from build123d import *
from build123d.topology import SkipClean

# Parameters (mm, degrees)
SKETCH1_W                = 105
SKETCH1_H                = 105
SKETCH1_W_2              = 94
SKETCH1_H_2              = 94
SKETCH1_W_3              = 65
SKETCH1_H_3              = 25
BOSS_EXTRUDE1_DEPTH      = 20
SKETCH2_W                = 65
SKETCH2_H                = 25
SKETCH2_W_2              = 94
SKETCH2_H_2              = 94
BOSS_EXTRUDE2_DEPTH      = 10
SKETCH3_W                = 57
SKETCH3_H                = 26.5
CUT_EXTRUDE1_DEPTH       = 20
SKETCH5_R                = 52.5
BOSS_EXTRUDE4_DEPTH      = 20
SKETCH8_R                = 48.5
CUT_EXTRUDE3_DEPTH       = 107.124926384
BOSS_EXTRUDE5_START      = -38
SKETCH9_R                = 2.5
BOSS_EXTRUDE5_DEPTH      = 12
SKETCH4_R                = 2.5
BOSS_EXTRUDE6_DEPTH      = 20
SKETCH10_W               = 15.5
SKETCH10_H               = 26.597794237
CUT_EXTRUDE4_DEPTH       = 20
BOSS_EXTRUDE8_START      = -45
SKETCH11_R               = 2.5
BOSS_EXTRUDE8_DEPTH      = 15
BOSS_EXTRUDE7_DEPTH      = 20
SKETCH16_R               = 2.5
BOSS_EXTRUDE9_DEPTH      = 30
CUT_EXTRUDE5_START       = -8
CUT_EXTRUDE5_DEPTH       = 8
SKETCH18_R               = 2.5
BOSS_EXTRUDE10_DEPTH     = 12
CUT_EXTRUDE12_DEPTH      = 18
CUT_EXTRUDE12_DEPTH_BACK = 24
CUT_EXTRUDE13_DEPTH      = 15


# Read off the part's stored shape, not the designer's step: Boss-Extrude7
with BuildPart() as part:
    # Sketch1 → Boss-Extrude1 (new body)
    # profile 1 of 2: a face of its own
    with BuildSketch(Plane.XY):
        Rectangle(SKETCH1_W, SKETCH1_H)
        Rectangle(SKETCH1_W_2, SKETCH1_H_2, mode=Mode.SUBTRACT)
    # profile 2 of 2: a face of its own
    with BuildSketch(Plane.XY):
        with Locations((0, -65)):
            Rectangle(SKETCH1_W_3, SKETCH1_H_3)
    extrude(amount=BOSS_EXTRUDE1_DEPTH)

    # Sketch2 → Boss-Extrude2 (add)
    # profile 1 of 3: a face of its own
    with BuildSketch(Plane.XY.offset(20)):
        with Locations((0, -65)):
            Rectangle(SKETCH2_W, SKETCH2_H)
    # profile 2 of 3: a face of its own
    with BuildSketch(Plane.XY.offset(20)):
        Polygon((52.5, 52.5), (-52.5, 52.5), (-52.5, -52.5), (-32.5, -52.5), (32.5, -52.5), (52.5, -52.5), align=None)
        Rectangle(SKETCH2_W_2, SKETCH2_H_2, mode=Mode.SUBTRACT)
    # profile 3 of 3: a face of its own
    with BuildSketch(Plane.XY.offset(20)):
        Rectangle(SKETCH2_W_2, SKETCH2_H_2)
    extrude(amount=BOSS_EXTRUDE2_DEPTH)

    # Sketch3 → Cut-Extrude1 (cut)
    with BuildSketch(Plane(origin=(0, 0, 0), x_dir=(-1, 0, 0), z_dir=(0, 0, -1))):
        with Locations((0, -60.25)):
            Rectangle(SKETCH3_W, SKETCH3_H)
    extrude(amount=-CUT_EXTRUDE1_DEPTH, mode=Mode.SUBTRACT)

    # Sketch5 → Boss-Extrude4 (add)
    with BuildSketch(Plane.XY.offset(30)):
        Circle(SKETCH5_R)
    extrude(amount=BOSS_EXTRUDE4_DEPTH)

    # Sketch8 → Cut-Extrude3 (cut, through all)
    with BuildSketch(Plane.XY.offset(50)):
        Circle(SKETCH8_R)
    extrude(amount=-CUT_EXTRUDE3_DEPTH, mode=Mode.SUBTRACT)

    # Sketch9 → Boss-Extrude5 (add)
    # profile 1 of 3: a face of its own
    with BuildSketch(Plane.XY.offset(50).offset(BOSS_EXTRUDE5_START)):
        with BuildLine():
            Line((57.5, 6.5), (48.5, 6.5))
            Line((48.5, 6.5), (48.5, -6.5))
            Line((48.5, -6.5), (57.5, -6.5))
            ThreePointArc((57.5, -6.5), (64, 0), (57.5, 6.5))
        make_face()
        with Locations((57.5, 0)):
            Circle(SKETCH9_R, mode=Mode.SUBTRACT)
    # profile 2 of 3: a face of its own
    with BuildSketch(Plane.XY.offset(50).offset(BOSS_EXTRUDE5_START)):
        with BuildLine():
            Line((-57.5, 6.5), (-48.5, 6.5))
            Line((-48.5, 6.5), (-48.5, -6.5))
            Line((-48.5, -6.5), (-57.5, -6.5))
            ThreePointArc((-57.5, -6.5), (-64, 0), (-57.5, 6.5))
        make_face()
        with Locations((-57.5, 0)):
            Circle(SKETCH9_R, mode=Mode.SUBTRACT)
    # profile 3 of 3: a face of its own
    with BuildSketch(Plane.XY.offset(50).offset(BOSS_EXTRUDE5_START)):
        with BuildLine():
            Line((-6.5, 57.5), (-6.5, 48.5))
            Line((-6.5, 48.5), (6.5, 48.5))
            Line((6.5, 48.5), (6.5, 57.5))
            ThreePointArc((6.5, 57.5), (0, 64), (-6.5, 57.5))
        make_face()
        with Locations((0, 57.5)):
            Circle(SKETCH9_R, mode=Mode.SUBTRACT)
    extrude(amount=-BOSS_EXTRUDE5_DEPTH)

    # Sketch4 → Boss-Extrude6 (add)
    with BuildSketch(Plane(origin=(0, 0, 0), x_dir=(-1, 0, 0), z_dir=(0, 0, -1))):
        with BuildLine():
            Line((-32.5, -64), (-32.5, -77.5))
            Line((-32.5, -77.5), (32.5, -77.5))
            Line((32.5, -77.5), (32.5, -64))
            Line((32.5, -64), (37.5, -64))
            ThreePointArc((37.5, -64), (42.096194078, -62.096194078), (44, -57.5))
            Line((44, -57.5), (44, -52.5))
            Line((44, -52.5), (52.5, -52.5))
            Line((52.5, -52.5), (52.021296507, -7.073521736))
            ThreePointArc((52.021296507, -7.073521736), (49.206713639, -18.301621043), (44, -28.640006983))
            Line((44, -28.640006983), (44, -20.402205763))
            ThreePointArc((44, -20.402205763), (0, -48.5), (-44, -20.402205763))
            Line((-44, -20.402205763), (-44, -28.640006983))
            ThreePointArc((-44, -28.640006983), (-50.330159944, -14.937369246), (-52.5, 0))
            Line((-52.5, 0), (-52.5, -52.5))
            Line((-52.5, -52.5), (-44, -52.5))
            Line((-44, -52.5), (-44, -57.5))
            ThreePointArc((-44, -57.5), (-42.096194078, -62.096194078), (-37.5, -64))
            Line((-37.5, -64), (-32.5, -64))
        make_face()
        with Locations((-37.5, -57.5)):
            Circle(SKETCH4_R, mode=Mode.SUBTRACT)
        with Locations((37.5, -57.5)):
            Circle(SKETCH4_R, mode=Mode.SUBTRACT)
    extrude(amount=-BOSS_EXTRUDE6_DEPTH)

    # Sketch10 → Cut-Extrude4 (cut)
    with BuildSketch(Plane(origin=(0, 0, 0), x_dir=(-1, 0, 0), z_dir=(0, 0, -1))):
        with Locations((-36.25, -33.701102881)):
            Rectangle(SKETCH10_W, SKETCH10_H)
        with Locations((37.754368076, -33.701102881)):
            Rectangle(SKETCH10_W, SKETCH10_H)
    extrude(amount=-CUT_EXTRUDE4_DEPTH, mode=Mode.SUBTRACT)

    # Sketch11 → Boss-Extrude8 (add)
    with BuildSketch(Plane.XY.offset(50).offset(BOSS_EXTRUDE8_START)):
        with Locations(Location((-37.5, -57.5, 0), (0, 0, 180))):
            Circle(SKETCH11_R)
        with Locations(Location((37.5, -57.5, 0), (0, 0, 180))):
            Circle(SKETCH11_R)
    extrude(amount=BOSS_EXTRUDE8_DEPTH)

    # Boss-Extrude7 outline → Boss-Extrude7 (add)
    with SkipClean():  # the faces are left unmerged after this step: merging them gives an invalid solid
        with BuildSketch(Plane.XY):
            with BuildLine():
                ThreePointArc((-30.004368076, -38.104958947), (-40.659489217, -26.439665971), (-47, -11.968709204))
                Line((-47, -11.968709204), (-47, -23.393375131))
                ThreePointArc((-47, -23.393375131), (-46.273225972, -24.79997093), (-45.504368076, -26.18401203))
                Line((-45.504368076, -26.18401203), (-45.504368076, -47))
                Line((-45.504368076, -47), (-30.004368076, -47))
                Line((-30.004368076, -47), (-30.004368076, -38.104958947))
            make_face()
            with BuildLine():
                Line((47, -23.393375131), (47, -11.968709204))
                ThreePointArc((47, -11.968709204), (40.137662704, -27.225319699), (28.5, -39.242833741))
                Line((28.5, -39.242833741), (28.5, -47))
                Line((28.5, -47), (44, -47))
                Line((44, -47), (44, -28.640006983))
                ThreePointArc((44, -28.640006983), (45.575561285, -26.059896653), (47, -23.393375131))
            make_face()
        extrude(amount=BOSS_EXTRUDE7_DEPTH)

    # Sketch16 → Boss-Extrude9 (add)
    with SkipClean():  # the faces are left unmerged after this step: merging them gives an invalid solid
        with BuildSketch(Plane.XY.offset(20)):
            with BuildLine():
                Line((-6.5, -57.496065111), (-6.5, -52.096065111))
                ThreePointArc((-6.5, -52.096065111), (0, -52.5), (6.5, -52.096065111))
                Line((6.5, -52.096065111), (6.5, -57.496065111))
                ThreePointArc((6.5, -57.496065111), (0, -63.996065111), (-6.5, -57.496065111))
            make_face()
            with Locations(Location((0, -57.496065111, 0), (0, 0, 180))):
                Circle(SKETCH16_R, mode=Mode.SUBTRACT)
        extrude(amount=BOSS_EXTRUDE9_DEPTH)

    # Sketch17 → Cut-Extrude5 (cut)
    with SkipClean():  # the faces are left unmerged after this step: merging them gives an invalid solid
        with BuildSketch(Plane.XY.offset(20).offset(CUT_EXTRUDE5_START)):
            with BuildLine():
                Line((32.5, -64), (32.5, -52.5))
                Line((32.5, -52.5), (44, -52.5))
                Line((44, -52.5), (44, -57.5))
                ThreePointArc((44, -57.5), (42.096194078, -62.096194078), (37.5, -64))
                Line((37.5, -64), (32.5, -64))
            make_face()
            with BuildLine():
                Line((-44, -52.5), (-32.5, -52.5))
                Line((-32.5, -52.5), (-32.5, -64))
                Line((-32.5, -64), (-37.5, -64))
                ThreePointArc((-37.5, -64), (-42.096194078, -62.096194078), (-44, -57.5))
                Line((-44, -57.5), (-44, -52.5))
            make_face()
        extrude(amount=CUT_EXTRUDE5_DEPTH, mode=Mode.SUBTRACT)

    # Sketch18 → Boss-Extrude10 (add)
    # profile 1 of 3: a face of its own
    with SkipClean():  # the faces are left unmerged after this step: merging them gives an invalid solid
        with BuildSketch(Plane.XY.offset(50)):
            with BuildLine():
                Line((-57.5, 6.5), (-52.096065111, 6.5))
                ThreePointArc((-52.096065111, 6.5), (-52.5, 0), (-52.096065111, -6.5))
                Line((-52.096065111, -6.5), (-57.5, -6.5))
                ThreePointArc((-57.5, -6.5), (-64, 0), (-57.5, 6.5))
            make_face()
            with Locations((-57.5, 0)):
                Circle(SKETCH18_R, mode=Mode.SUBTRACT)
        # profile 2 of 3: a face of its own
        with BuildSketch(Plane.XY.offset(50)):
            with BuildLine():
                Line((52.096065111, 6.5), (57.5, 6.5))
                ThreePointArc((57.5, 6.5), (64, 0), (57.5, -6.5))
                Line((57.5, -6.5), (52.096065111, -6.5))
                ThreePointArc((52.096065111, -6.5), (52.5, 0), (52.096065111, 6.5))
            make_face()
            with Locations((57.5, 0)):
                Circle(SKETCH18_R, mode=Mode.SUBTRACT)
        # profile 3 of 3: a face of its own
        with BuildSketch(Plane.XY.offset(50)):
            with BuildLine():
                Line((-6.5, 57.5), (-6.5, 52.096065111))
                ThreePointArc((-6.5, 52.096065111), (0, 52.5), (6.5, 52.096065111))
                Line((6.5, 52.096065111), (6.5, 57.5))
                ThreePointArc((6.5, 57.5), (0, 64), (-6.5, 57.5))
            make_face()
            with Locations((0, 57.5)):
                Circle(SKETCH18_R, mode=Mode.SUBTRACT)
        extrude(amount=-BOSS_EXTRUDE10_DEPTH)

    # Sketch19 → Cut-Extrude12 (cut, two sides: drawn at the far end of the back side and taken through both)
    with SkipClean():  # the faces are left unmerged after this step: merging them gives an invalid solid
        with BuildSketch(Plane(origin=(0, 0, 0), x_dir=(-1, 0, 0), z_dir=(0, 0, -1)).offset(-CUT_EXTRUDE12_DEPTH_BACK)):
            with BuildLine():
                Line((-6.5, -57.496065111), (-6.5, -46.382922992))
                ThreePointArc((-6.5, -46.382922992), (0, -46.836156389), (6.5, -46.382922992))
                Line((6.5, -46.382922992), (6.5, -57.496065111))
                ThreePointArc((6.5, -57.496065111), (0, -63.996065111), (-6.5, -57.496065111))
            make_face()
        extrude(amount=CUT_EXTRUDE12_DEPTH + CUT_EXTRUDE12_DEPTH_BACK, mode=Mode.SUBTRACT)

    # Sketch20 → Cut-Extrude13 (cut)
    with SkipClean():  # the faces are left unmerged after this step: merging them gives an invalid solid
        with BuildSketch(Plane(origin=(0, 0, 24), x_dir=(-1, 0, 0), z_dir=(0, 0, -1))):
            with BuildLine():
                Line((4.5, -57.496065111), (4.5, -48.290785871))
                ThreePointArc((4.5, -48.290785871), (0, -48.5), (-4.5, -48.290785871))
                Line((-4.5, -48.290785871), (-4.5, -57.496065111))
                ThreePointArc((-4.5, -57.496065111), (0, -61.996065111), (4.5, -57.496065111))
            make_face()
        extrude(amount=-CUT_EXTRUDE13_DEPTH, mode=Mode.SUBTRACT)


solid = part.part
Part model, mm, in its own coordinate system. A direction names the side the tool comes from. Give positions to 0.01 mm unless a question says otherwise; leave off trailing zeros. Write each loop counter-clockwise with the first axis right and the second up, starting at its lowest first coordinate (ties: lowest second). Pieces come first, ordered by that corner, then holes.
1) Cut at B-B on z = 14.5. Write the cut outline in (x, y).
Resolved:
outline: (-52.5, -52.5) - (-32.5, -52.5) - (-32.5, -77.5) - (32.5, -77.5) - (32.5, -52.5) - (52.5, -52.5) - (52.5, 52.5) - (-52.5, 52.5) - close; hole (-47, 11.97) arc R48.5 ccw to (-6.5, -48.06) - (-6.5, -57.5) arc R6.5 ccw to (6.5, -57.5) - (6.5, -48.06) arc R48.5 ccw to (47, 11.97) - (47, 47) - (11.97, 47) arc R48.5 ccw to (-11.97, 47) - (-47, 47) - close
2) Two-plate mould, pull along X, no slides. Class faces 4 (the face through (-6.5, -55, 40)), 5 (the face through (55, 6.5, 44)), 6 (the face through (-4.5, -53, 31)): released by +X, released by -X, zero draft, split by the parting line, or undercut.
Resolved:
face 4: released by -X
face 5: zero draft
face 6: undercut
3) Which spindle directions (+Z, -Z, +X, -X, +Y, -Y) get a long thin tool onto all of the face, cutting with end or side? Do faces 1 (the face through (58, -3, 12)), 2 (the face through (44, -55, 6)), 3 (the face through (-2, 60, 12)). Say none if no direction does.
Resolved:
face 1: +X, +Y, -Y
face 2: +Z, -Z, +X, -Y
face 3: +X, -X, +Y
4) Cut at A-A on z = 45.5. Write the cut outline in (x, y), then the cut area to 3 significant figures.
Resolved:
outline: (-57.5, -6.5) - (-52.1, -6.5) arc R52.5 ccw to (-6.5, -52.1) - (-6.5, -57.5) arc R6.5 ccw to (6.5, -57.5) - (6.5, -52.1) arc R52.5 ccw to (52.1, -6.5) - (57.5, -6.5) arc R6.5 ccw to (57.5, 6.5) - (52.1, 6.5) arc R52.5 ccw to (6.5, 52.1) - (6.5, 57.5) arc R6.5 ccw to (-6.5, 57.5) - (-6.5, 52.1) arc R52.5 ccw to (-52.1, 6.5) - (-57.5, 6.5) arc R6.5 ccw to start; hole circle Ø5 at (-57.5, 0); hole circle Ø97 at (0, 0); hole circle Ø5 at (0, -57.5); hole circle Ø5 at (0, 57.5); hole circle Ø5 at (57.5, 0)
area: 1,720 mm2
5) Cut at D-D on y = 31. Write the cut outline in (x, z), then the cut area to 3 significant figures.
Resolved:
outline: (-52.5, 0) - (-47, 0) - (-47, 20) - (-37.3, 20) - (-37.3, 50) - (-42.37, 50) - (-42.37, 30) - (-52.5, 30) - close; (37.3, 20) - (47, 20) - (47, 0) - (52.5, 0) - (52.5, 30) - (42.37, 30) - (42.37, 50) - (37.3, 50) - close
area: 727 mm2
6) Probe L1, parallel to Y at x = 0, z = 47.5; L2, parallel to Y at x = 57.5, z = 9; L3, parallel to Y at x = 0, z = 6. List the from-to ranges inside material, lowest first.
Resolved:
L1: y = -64 to -60, -55 to -48.5, 48.5 to 55, 60 to 64
L2: y = -6.5 to -2.5, 2.5 to 6.5
L3: y = -77.5 to -64, 48.5 to 55, 60 to 64
7) Pin check, flat tips, straight feed: pin 1 (1.5 mm diameter, centred on y = 38, z = 37.5, fed in from +X); pin 2 (6 mm diameter, centred on y = 24.5, z = 20, fed in from +X); pin 3 (1.5 mm diameter, centred on x = 55, z = 6.5, fed in from +Y). Stop position of each tip, or through.
Resolved:
pin 1: stops at x = 37
pin 2: stops at x = 52.5
pin 3: stops at y = 6.5
8) Cut at C-C on y = -33.5. Write the cut outline in (x, z).
Resolved:
outline: (-52.5, 0) - (-35.07, 0) - (-35.07, 50) - (-40.42, 50) - (-40.42, 30) - (-52.5, 30) - close; (35.07, 0) - (52.5, 0) - (52.5, 30) - (40.42, 30) - (40.42, 50) - (35.07, 50) - close
